from build123d import *

# Parameters (mm, degrees)
SKETCH1_W                = 8
SKETCH1_H                = 8
BOSS_EXTRUDE1_DEPTH      = 8
FILLET1_R                = 0.9
BOSS_EXTRUDE2_DEPTH      = 2
BOSS_EXTRUDE2_DEPTH_BACK = 10
SKETCH2_R                = 2
SKETCH4_R                = 2
BOSS_EXTRUDE6_DEPTH      = 10


with BuildPart() as part:
    # Sketch1 → Boss-Extrude1 (new body)
    with BuildSketch(Plane.XY):
        Rectangle(SKETCH1_W, SKETCH1_H)
    extrude(amount=BOSS_EXTRUDE1_DEPTH)

    # Fillet1
    fillet1_edges = [part.edges().sort_by_distance(p)[0] for p in [
        (4, 0, 8),
        (0, 4, 8),
        (-4, 0, 8),
        (0, 4, 0),
        (4, 0, 0),
        (0, -4, 0),
        (-4, 0, 0),
        (0, -4, 8),
        (-4, 4, 4),
        (4, 4, 4),
        (4, -4, 4),
        (-4, -4, 4),
    ]]
    fillet(fillet1_edges, radius=FILLET1_R)

    # Sketch2 → Boss-Extrude2 (add, two sides: drawn at the far end of the back side and taken through both)
    with BuildSketch(Plane.XY.offset(8).offset(-BOSS_EXTRUDE2_DEPTH_BACK)):
        Circle(SKETCH2_R)
    extrude(amount=BOSS_EXTRUDE2_DEPTH + BOSS_EXTRUDE2_DEPTH_BACK)

    # Sketch4 → Boss-Extrude6 (add, symmetric)
    with BuildSketch(Plane(origin=(0, 0, 0), x_dir=(0, 0, -1), z_dir=(1, 0, 0))):
        with Locations(Location((-3.978609227, 0, 0), (0, 0, 180))):
            Circle(SKETCH4_R)
    extrude(amount=BOSS_EXTRUDE6_DEPTH, both=True)


solid = part.part
Work out the finished part from the listing and answer in its coordinate system (mm). A direction names the side the tool comes from. Coordinates: 2 decimals unless noted, no trailing zeros. Loops run counter-clockwise (first coordinate to the right, second up) from the corner with the lowest first, then second, coordinate; pieces in that order, holes last. Notation, with made-up numbers: M 69.5,-14 L 113.5,-14 A31 ccw 113.5,13 Z; hole C 70.25,-1 d5. An arc over 180 degrees is marked long. Answer in a Markdown table with one row per item. Add a question column.
1. Find section B-B, the plane y = 0. Write down the section's boundary in (x, z).
2. Consider L1, parallel to X at y = -2.5, z = 7; L2, parallel to Z at x = 3.25, y = 0.25; L3, parallel to Y at x = -4.25, z = 5.25. Determine where each line is inside the solid, lowest interval first.
3. A tool of negligible diameter and unlimited length cuts with its end or side. For faces 1 (the cylindrical face through (0, -2, 9)), 2 (the flat face through (-1, 2, 0)), 3 (the cylindrical face through (-6.96, -0.09, 1.98)), from which of +Z, -Z, +X, -X, +Y, -Y can it reach the whole face along a straight path? Write none if from no direction.
4. Find section D-D, the plane z = 3.5. Write down the section's boundary in (x, y), then the cut area to 3 significant figures.
5. Flat-ended cylindrical pins translate along their axes: P1, Ø1.5, axis at y = 1.5, z = 7, coming from the -X side; P2, Ø1, axis at x = -5, z = 5.5, coming from the -Y side; P3, Ø2, axis at x = -0.5, y = 2, coming from the -Z side. Find the tip coordinate at first contact, or state that the pin passes through.
6. Find section A-A, the plane x = 0. Write down the section's boundary in (y, z).
7. Find section C-C, the plane z = 1.75. Write down the section's boundary in (x, y).
Reported:
| question | item | result |
|---|---|---|
| 1 | outline | M -10,1.98 L -4,1.98 L -4,0.9 A0.9 ccw -3.1,0 L -2,0 L -2,-2 L 2,-2 L 2,0 L 3.1,0 A0.9 ccw 4,0.9 L 4,1.98 L 10,1.98 L 10,5.98 L 4,5.98 L 4,7.1 A0.9 ccw 3.1,8 L 2,8 L 2,10 L -2,10 L -2,8 L -3.1,8 A0.9 ccw -4,7.1 L -4,5.98 L -10,5.98 Z |
| 2 | L1 | x = -4 to 4 |
| 2 | L2 | z = 0.01 to 7.99 |
| 2 | L3 | y = -1.54 to 1.54 |
| 3 | face 1 | +Z |
| 3 | face 2 | -Z |
| 3 | face 3 | -X |
| 4 | outline | M -10,-1.94 L -4,-1.94 L -4,-3.1 A0.9 ccw -3.1,-4 L 3.1,-4 A0.9 ccw 4,-3.1 L 4,-1.94 L 10,-1.94 L 10,1.94 L 4,1.94 L 4,3.1 A0.9 ccw 3.1,4 L -3.1,4 A0.9 ccw -4,3.1 L -4,1.94 L -10,1.94 Z |
| 4 | area | 110 mm^2 |
| 5 | P1 | stops at x = -4 |
| 5 | P2 | stops at y = -1.72 |
| 5 | P3 | stops at z = -2 |
| 6 | outline | M -4,0.9 A0.9 ccw -3.1,0 L -2,0 L -2,-2 L 2,-2 L 2,0 L 3.1,0 A0.9 ccw 4,0.9 L 4,7.1 A0.9 ccw 3.1,8 L 2,8 L 2,10 L -2,10 L -2,8 L -3.1,8 A0.9 ccw -4,7.1 Z |
| 7 | outline | M -4,-3.1 A0.9 ccw -3.1,-4 L 3.1,-4 A0.9 ccw 4,-3.1 L 4,3.1 A0.9 ccw 3.1,4 L -3.1,4 A0.9 ccw -4,3.1 Z |
